Could you check a few things on this model? Use its own coordinates, in mm. A direction names the side the tool comes from. Give positions to 0.01 mm unless a question says otherwise; leave off trailing zeros. Write each loop counter-clockwise with the first axis right and the second up, starting at its lowest first coordinate (ties: lowest second). Pieces come first, ordered by that corner, then holes. Notation, with made-up numbers: M -24.5,66.25 L 1.5,66.25 A14 cw 1.5,83.25 Z; hole C 45,83.25 d10. An arc over 180 degrees is marked long. Answer as a JSON object with one key per item and string values. Group by question number.
```python
from build123d import *

# Parameters (mm, degrees)
SKETCH1_R           = 32.5
BOSS_EXTRUDE1_DEPTH = 56
CUT_EXTRUDE4_START  = -54
SKETCH6_R           = 32.5
SKETCH6_R_2         = 22.5
CUT_EXTRUDE4_DEPTH  = 52
SKETCH2_R           = 1.5
CUT_EXTRUDE2_DEPTH  = 73.446532008
SHELL1_OUTLINE_R    = 20.5
SHELL1_DEPTH        = 56


# Read off the part's stored shape, not the designer's step: Shell1
with BuildPart() as part:
    # Sketch1 → Boss-Extrude1 (new body)
    with BuildSketch(Plane(origin=(0, 0, 0), x_dir=(1, 0, 0), z_dir=(0, 1, 0))):
        with Locations(Location((0, 0, 0), (0, 0, 270))):
            Circle(SKETCH1_R)
    extrude(amount=BOSS_EXTRUDE1_DEPTH)

    # Sketch6 → Cut-Extrude4 (cut)
    with BuildSketch(Plane(origin=(0, 56, 0), x_dir=(1, 0, 0), z_dir=(0, 1, 0)).offset(CUT_EXTRUDE4_START)):
        with Locations(Location((0, 0, 0), (0, 0, 270))):
            Circle(SKETCH6_R)
        with Locations(Location((0, 0, 0), (0, 0, 270))):
            Circle(SKETCH6_R_2, mode=Mode.SUBTRACT)
    extrude(amount=CUT_EXTRUDE4_DEPTH, mode=Mode.SUBTRACT)

    # Sketch2 → Cut-Extrude2 (cut, through all)
    with BuildSketch(Plane(origin=(0, 56, 0), x_dir=(1, 0, 0), z_dir=(0, 1, 0))):
        with Locations(Location((0, 29, 0), (0, 0, 270))):
            Circle(SKETCH2_R)
        with Locations(Location((-25.11473671, -14.5, 0), (0, 0, 270))):
            Circle(SKETCH2_R)
        with Locations(Location((25.11473671, -14.5, 0), (0, 0, 270))):
            Circle(SKETCH2_R)
    extrude(amount=-CUT_EXTRUDE2_DEPTH, mode=Mode.SUBTRACT)

    # Shell1 outline → Shell1 (cut)
    with BuildSketch(Plane(origin=(0, 0, 0), x_dir=(1, 0, 0), z_dir=(0, 1, 0))):
        Circle(SHELL1_OUTLINE_R)
    extrude(amount=SHELL1_DEPTH, mode=Mode.SUBTRACT)


solid = part.part
```
1) Please list where these lines run through material, in increasing order: line 1 along Y through (x, z) = (-14, -20.5); line 2 along Z through (x, y) = (6, 17.5); line 3 along Z through (x, y) = (-4, 13.5). Write a range as from..to.
2) If we section it at D-D, the plane z = 14.5: Give the number of separate pieces and of enclosed holes in the cut face, plus the area to 3 significant figures.
3) If we section it at C-C, the plane x = -7: List the corners of the cut face in (y, z) for me, plus the area to 3 significant figures.
4) If we section it at B-B, the plane z = 0: List the corners of the cut face in (x, y) for me.
5) We'd pull the mould along Y, two halves only. Please class faces 3 (the cylindrical face through (-26.03, 55.01, 13.31)), 4 (the cylindrical face through (-8.618, 27.636, 20.784)), 5 (the flat face through (0, 0, 21)), 6 (the flat face through (22, 2, 7)): released by +Y, released by -Y, zero draft, split by the parting line, or undercut.
6) For faces 1 (the flat face through (22, 54, 7)), 2 (the cylindrical face through (0.07, 55.01, -30.5)), which set-ups out of +Z, -Z, +X, -X, +Y, -Y let a thin tool reach every point of the face, with its end or its side?
7) I'm going to push flat-ended pins straight in: pin 1 (1 mm diameter, centred on y = 7.5, z = -13.5, fed in from -X); pin 2 (4 mm diameter, centred on x = 0, z = -29, fed in from -Y); pin 3 (6 mm diameter, centred on y = 11, z = -16, fed in from +X); pin 4 (6 mm diameter, centred on x = 5, y = 7.5, fed in from +Z). Where does each tip first touch, or does it pass through?
8) If we section it at A-A, the plane x = 0: List the corners of the cut face in (y, z) for me.
Taken from the geometry:
{
 "1": {"line 1": "0..2, 54..56", "line 2": "-21.69..-19.6, 19.6..21.69", "line 3": "-22.14..-20.11, 20.11..22.14"},
 "2": {"separate pieces": "6", "enclosed holes": "0", "area": "375 mm²"},
 "3": {"outline": "M 0,-31.74 L 2,-31.74 L 2,-21.38 L 54,-21.38 L 54,-31.74 L 56,-31.74 L 56,-19.27 L 0,-19.27 Z; M 0,19.27 L 56,19.27 L 56,31.74 L 54,31.74 L 54,21.38 L 2,21.38 L 2,31.74 L 0,31.74 Z", "area": "320 mm²"},
 "4": {"outline": "M -32.5,0 L -20.5,0 L -20.5,56 L -32.5,56 L -32.5,54 L -22.5,54 L -22.5,2 L -32.5,2 Z; M 20.5,0 L 32.5,0 L 32.5,2 L 22.5,2 L 22.5,54 L 32.5,54 L 32.5,56 L 20.5,56 Z"},
 "5": {"face 3": "zero draft", "face 4": "undercut", "face 5": "released by -Y", "face 6": "undercut"},
 "6": {"face 1": "none", "face 2": "+Y, -Y"},
 "7": {"pin 1": "x = -18.36", "pin 2": "y = 0", "pin 3": "x = 18.36", "pin 4": "z = 22.41"},
 "8": {"outline": "M 0,-32.5 L 2,-32.5 L 2,-30.5 L 0,-30.5 Z; M 0,-27.5 L 2,-27.5 L 2,-22.5 L 54,-22.5 L 54,-27.5 L 56,-27.5 L 56,-20.5 L 0,-20.5 Z; M 0,20.5 L 56,20.5 L 56,32.5 L 54,32.5 L 54,22.5 L 2,22.5 L 2,32.5 L 0,32.5 Z; M 54,-32.5 L 56,-32.5 L 56,-30.5 L 54,-30.5 Z"}
}
